Geometry: final body of the model. Coordinates: model frame, mm. A direction names the side the tool comes from. Coordinates: 2 decimals unless noted, no trailing zeros. Write each loop counter-clockwise with the first axis right and the second up, starting at its lowest first coordinate (ties: lowest second). Pieces come first, ordered by that corner, then holes.
from build123d import *

# Parameters (mm, degrees)
SKETCH1_W                                           = 20
SKETCH1_H                                           = 55
BOSS_EXTRUDE1_DEPTH                                 = 20
SKETCH2_R                                           = 4
CUT_EXTRUDE1_DEPTH                                  = 10
SKETCH3_W                                           = 20
SKETCH3_H                                           = 20
CUT_EXTRUDE2_DEPTH                                  = 10
CBORE_FOR_M3_HEX_SOCKET_HEAD_CAP_SCREW1_D           = 3.4
CBORE_FOR_M3_HEX_SOCKET_HEAD_CAP_SCREW1_CBORE_D     = 6.5
CBORE_FOR_M3_HEX_SOCKET_HEAD_CAP_SCREW1_CBORE_DEPTH = 3.4
FILLET2_R                                           = 5
SKETCH9_R                                           = 2.25
CUT_EXTRUDE5_DEPTH                                  = 40.449334595
CUT_EXTRUDE6_DEPTH                                  = 4


with BuildPart() as part:
    # Sketch1 → Boss-Extrude1 (new body)
    with BuildSketch(Plane(origin=(0, 0, 0), x_dir=(1, 0, 0), z_dir=(0, 1, 0))):
        Rectangle(SKETCH1_W, SKETCH1_H)
    extrude(amount=BOSS_EXTRUDE1_DEPTH)

    # Sketch2 → Cut-Extrude1 (cut)
    with BuildSketch(Plane(origin=(0, 20, 0), x_dir=(1, 0, 0), z_dir=(0, 1, 0))):
        with Locations(Location((-3, 0, 0), (0, 0, 270))):
            Circle(SKETCH2_R)
    extrude(amount=-CUT_EXTRUDE1_DEPTH, mode=Mode.SUBTRACT)

    # Sketch3 → Cut-Extrude2 (cut)
    with BuildSketch(Plane(origin=(0, 20, 0), x_dir=(1, 0, 0), z_dir=(0, 1, 0))):
        with Locations((0, -17.5)):
            Rectangle(SKETCH3_W, SKETCH3_H)
        with Locations((0, 17.5)):
            Rectangle(SKETCH3_W, SKETCH3_H)
    extrude(amount=-CUT_EXTRUDE2_DEPTH, mode=Mode.SUBTRACT)

    # CBORE for M3 Hex Socket Head Cap Screw1 (through all)
    with Locations(Plane(origin=(0, 10, 0), x_dir=(1, 0, 0), z_dir=(0, 1, 0))):
        with Locations((0, -15.5), (0, 15.5)):
            CounterBoreHole(CBORE_FOR_M3_HEX_SOCKET_HEAD_CAP_SCREW1_D / 2, CBORE_FOR_M3_HEX_SOCKET_HEAD_CAP_SCREW1_CBORE_D / 2, CBORE_FOR_M3_HEX_SOCKET_HEAD_CAP_SCREW1_CBORE_DEPTH)

    # Fillet2
    fillet2_edges = [part.edges().sort_by_distance(p)[0] for p in [
        (-10, 15, 7.5),
        (10, 15, 7.5),
        (-10, 15, -7.5),
        (10, 15, -7.5),
    ]]
    fillet(fillet2_edges, radius=FILLET2_R)

    # Sketch9 → Cut-Extrude5 (cut, through all)
    with BuildSketch(Plane.ZY.offset(10)):
        with Locations((-21, 5)):
            Circle(SKETCH9_R)
        with Locations((21, 5)):
            Circle(SKETCH9_R)
    extrude(amount=-CUT_EXTRUDE5_DEPTH, mode=Mode.SUBTRACT)

    # Sketch10 → Cut-Extrude6 (cut)
    with BuildSketch(Plane(origin=(10, 0, 0), x_dir=(0, 0, -1), z_dir=(1, 0, 0))):
        Polygon((-16.958548116, 5), (-18.979274058, 8.5), (-23.020725942, 8.5), (-25.041451884, 5), (-23.020725942, 1.5), (-18.979274058, 1.5), align=None)
        Polygon((16.958548116, 5), (18.979274058, 1.5), (23.020725942, 1.5), (25.041451884, 5), (23.020725942, 8.5), (18.979274058, 8.5), align=None)
    extrude(amount=-CUT_EXTRUDE6_DEPTH, mode=Mode.SUBTRACT)


solid = part.part
Item 1: Section B-B, the plane y = 18.5. Output: boundary loops of the cut face in (x, z), plus the area to 3 significant figures.
Derived:
outline: (-10, -2.5) arc R5 ccw to (-5, -7.5) - (5, -7.5) arc R5 ccw to (10, -2.5) - (10, 2.5) arc R5 ccw to (5, 7.5) - (-5, 7.5) arc R5 ccw to (-10, 2.5) - close; hole circle Ø8 at (-3, 0)
area: 228 mm2
Item 2: Pin query (flat end, axial travel): pin 1 (2 mm diameter, centred on y = 4, z = -22.5, fed in from +X); pin 2 (2 mm diameter, centred on x = 0.5, z = 14, fed in from +Y); pin 3 (4 mm diameter, centred on x = 2, y = 14.5, fed in from +Z). Return the tip coordinate at first contact, or that it passes through.
Derived:
pin 1: stops at x = 6
pin 2: stops at y = 6.6
pin 3: stops at z = 7.5
Item 3: Set-up query: faces 4 (the flat face through (8, 6.8, 24)), 5 (the cylindrical face through (8.5, 14.93, -6.07)), 6 (the flat face through (1.4, 6.6, 16.9)). Return all of +Z, -Z, +X, -X, +Y, -Y with unobstructed straight access to the full face (end or side cutting, diameter ignored); none if empty.
Derived:
face 4: +X
face 5: -Z, +X, +Y
face 6: +Y
Item 4: Pull-direction query (Z, two-part tool) for faces 1 (the flat face through (1.4, 6.6, -14.1)), 2 (the cylindrical face through (-8.57, 14.93, -6)), 3 (the flat face through (0, 10, 20)); classes: released by +Z, released by -Z, zero draft, split by the parting line, or undercut.
Derived:
face 1: undercut
face 2: released by -Z
face 3: zero draft
Item 5: Section A-A, the plane z = -21. Output: boundary loops of the cut face in (x, y).
Derived:
outline: (-10, 0) - (10, 0) - (10, 1.5) - (6, 1.5) - (6, 2.75) - (-10, 2.75) - close; (-10, 7.25) - (6, 7.25) - (6, 8.5) - (10, 8.5) - (10, 10) - (-10, 10) - close
Item 6: Material intervals for probe 1 along Z at (x, y) = (0, 9.15); probe 2 along X at (y, z) = (4, -15.5); probe 3 along X at (y, z) = (13, 0), sorted ascending.
Derived:
probe 1: z = -27.5 to -18.75, -12.25 to 12.25, 18.75 to 27.5
probe 2: x = -10 to -1.7, 1.7 to 10
probe 3: x = -10 to -7, 1 to 10
Item 7: Section C-C, the plane x = 0. State how many separate pieces and enclosed holes the cut face has, plus the area to 3 significant figures.
Derived:
separate pieces: 3
enclosed holes: 2
area: 526 mm2
Item 8: Section D-D, the plane y = 5.75. Output: boundary loops of the cut face in (x, z).
Derived:
outline: (-10, -27.5) - (10, -27.5) - (10, -24.61) - (6, -24.61) - (6, -23.12) - (-10, -23.12) - close; (-10, -18.88) - (6, -18.88) - (6, -17.39) - (10, -17.39) - (10, 17.39) - (6, 17.39) - (6, 18.88) - (-10, 18.88) - close; (-10, 23.12) - (6, 23.12) - (6, 24.61) - (10, 24.61) - (10, 27.5) - (-10, 27.5) - close; hole circle Ø3.4 at (0, -15.5); hole circle Ø3.4 at (0, 15.5)
